For this review, take the finished solid that the model builds, in its own axes (mm). A direction names the side the tool comes from. Give positions to 0.01 mm unless a question says otherwise; leave off trailing zeros. Write each loop counter-clockwise with the first axis right and the second up, starting at its lowest first coordinate (ties: lowest second). Pieces come first, ordered by that corner, then holes. Notation, with made-up numbers: M 70,82 L 110,82 A19 cw 110,99 Z; hole C 57,40 d9. An arc over 180 degrees is marked long. Use one line per item in the form item = value. Start each with the question number.
Q1. Consider section A-A on z = 3.75. Write out the cut boundary in (x, y), and give its area (3 significant figures).
Q2. Tool access review of faces 1 (the cylindrical face through (-12.69, 24.397, 4.162)), 2 (the flat face through (1.05, -37.96, 0.99)), 3 (the cylindrical face through (34.9, -25.8, 1)): name each direction out of +Z, -Z, +X, -X, +Y, -Y from which nothing blocks a thin tool from reaching the whole face with its end or side.
Q3. Consider section C-C on z = 10.25. Write out the cut boundary in (x, y), and give its area (3 significant figures).
Q4. Clearance check with flat-ended pins moving along their axes: pin 1 Ø2.5 at (x, y) = (33.3, -12.68) entering from -Z; pin 2 Ø2 at (x, z) = (30, 1) entering from +Y; pin 3 Ø4 at (y, z) = (-53.5, 2.5) entering from -X; pin 4 Ø4 at (y, z) = (-42, 7) entering from +X. State where each tip first meets the part, or that it passes through.
Q5. Consider section D-D on x = 66.6. Write out the cut boundary in (y, z).
Q6. Consider section B-B on y = 0. Write out the cut boundary in (x, z), and give its area (3 significant figures).
Q7. Mouldability with a two-part tool opening along Y and no side actions: class faces 4 (the flat face through (34, -15, 0)), 5 (the cylindrical face through (28.35, -19.3, 0.99)) as released by +Y, released by -Y, zero draft, split by the parting line, or undercut.
Q8. For probe 1 along Y at (x, z) = (33.3, 1.25); probe 2 along Y at (x, z) = (0, 3.1); probe 3 along X at (y, z) = (-13, 4), list the stretches that pass through material, from the lowest coordinate up. Write a range as [from, to].
```python
from build123d import *

# Parameters (mm, degrees)
SKETCH_1_R          = 30
SKETCH_1_R_2        = 27.5
EXTRUDE_1_DEPTH     = 13
SKETCH_1_R_3        = 29.999999999999996
EXTRUDE_1_2_DEPTH   = 13
EXTRUDE_1_3_DEPTH   = 13
EXTRUDE_2_DEPTH     = 2
SKETCH_3_R          = 1.6500000000000017
SKETCH_3_R_2        = 1.5999999999999979
SKETCH_3_R_3        = 1.5999999999999985
SKETCH_3_R_4        = 1.6000000000000019
CUT_EXTRUDE_5_DEPTH = 132.10250765535577
FILLET_1_R          = 10


with BuildPart() as part:
    # Sketch 1 → Extrude 1 (new body)
    with BuildSketch(Plane.XY):
        with Locations(Location((0, 0, 0), (0, 0, 180))):
            Circle(SKETCH_1_R)
        with Locations(Location((0, 0, 0), (0, 0, 180))):
            Circle(SKETCH_1_R_2, mode=Mode.SUBTRACT)
    extrude(amount=EXTRUDE_1_DEPTH)



with BuildPart() as body_2:
    # Sketch 1 → Extrude 1 2 (new body)
    with BuildSketch(Plane.XY):
        with Locations(Location((66.6, 0, 0), (0, 0, 180))):
            Circle(SKETCH_1_R_3)
        with Locations(Location((66.6, 0, 0), (0, 0, 180))):
            Circle(SKETCH_1_R_2, mode=Mode.SUBTRACT)
    extrude(amount=EXTRUDE_1_2_DEPTH)


with BuildPart() as body_3:
    # Sketch 1 → Extrude 1 3 (new body)
    with BuildSketch(Plane.XY):
        with Locations(Location((33.30000000000001, -57.6772918920436, 0), (0, 0, 180))):
            Circle(SKETCH_1_R_3)
        with Locations(Location((33.30000000000001, -57.6772918920436, 0), (0, 0, 180))):
            Circle(SKETCH_1_R_2, mode=Mode.SUBTRACT)
    extrude(amount=EXTRUDE_1_3_DEPTH)


with BuildPart() as part_1:
    add(part.part)

    add(body_2.part)  # Extrude 2 merges body 2

    add(body_3.part)  # Extrude 2 merges body 3
    # Sketch 2 → Extrude 2 (add)
    with BuildSketch(Plane.XY):
        with BuildLine():
            Line((26.3198925252566, 18.070831312697457), (40.280107474743396, 18.070831312697457))
            ThreePointArc((40.280107474743396, 18.070831312697457), (42.3441853289733, 18.516758123597654), (44.04009212120862, 19.77499826802639))
            ThreePointArc((44.04009212120862, 19.77499826802639), (92.58076211353317, 15), (72.44569692050842, -29.424952464083248))
            ThreePointArc((72.44569692050842, -29.424952464083248), (70.50807559525407, -30.264530756395246), (69.08985272167097, -31.829111208097117))
            Line((69.08985272167097, -31.829111208097117), (62.10974524692759, -43.91901199664395))
            ThreePointArc((62.10974524692759, -43.91901199664395), (61.46389026628078, -45.92951925924603), (61.70560479929982, -48.027337695986766))
            ThreePointArc((61.70560479929982, -48.027337695986766), (33.300000000000004, -87.6772918920436), (4.894395200700185, -48.02733769598677))
            ThreePointArc((4.894395200700185, -48.02733769598677), (5.13610973371921, -45.92951925924604), (4.4902547530724135, -43.91901199664397))
            Line((4.4902547530724135, -43.91901199664397), (-2.489852721670984, -31.829111208097103))
            ThreePointArc((-2.489852721670984, -31.829111208097103), (-3.9080755952540875, -30.264530756395228), (-5.845696920508439, -29.42495246408323))
            ThreePointArc((-5.845696920508439, -29.42495246408323), (-25.980762113533153, 15.000000000000009), (22.55990787879137, 19.77499826802639))
            ThreePointArc((22.55990787879137, 19.77499826802639), (24.25581467102669, 18.516758123597654), (26.3198925252566, 18.070831312697457))
        make_face()
    extrude(amount=EXTRUDE_2_DEPTH)

    # Sketch 3 → Cut-Extrude 5 (cut, through all)
    with BuildSketch(Plane.XY):
        with Locations(Location((33.3, -19.225763964014533, 0), (0, 0, 180))):
            Circle(SKETCH_3_R)
        with Locations(Location((33.3, -12.678793774014526, 0), (0, 0, 180))):
            Circle(SKETCH_3_R_2)
        with Locations(Location((39.84697019, -19.225763964014533, 0), (0, 0, 180))):
            Circle(SKETCH_3_R_3)
        with Locations(Location((33.3, -25.772734154014536, 0), (0, 0, 180))):
            Circle(SKETCH_3_R_3)
        with Locations(Location((26.75302980999999, -19.225763964014533, 0), (0, 0, 180))):
            Circle(SKETCH_3_R_4)
    extrude(amount=CUT_EXTRUDE_5_DEPTH, mode=Mode.SUBTRACT)

    # Fillet 1
    # the kernel refuses this fillet: 10 mm, written as the material it takes off along each edge
    with BuildSketch(Plane(origin=(0, 0, 13), x_dir=(-1, 1.2e-16, 0), z_dir=(1.2e-16, 1, 0))) as fillet_1_piece_1:
        with BuildLine():
            CenterArc((37.5, -6.614378277661482), FILLET_1_R, 138.59037789072914, 41.409622109270856)
            Line((27.5, -6.614378277661482), (27.3, -6.614378277661482))
            Line((27.3, -6.614378277661482), (27.3, 0))
            Line((27.3, 0), (27.5, 0.1999999999999993))
            ThreePointArc((27.5, 0.1999999999999993), (28.75, 0.1999999999999993), (29.85, 0.1322875655532254))
            Line((29.85, 0.1322875655532254), (30, -3.55e-15))
        make_face()
    revolve(axis=Axis((0, 0, 13), (0, 0, 1)), mode=Mode.SUBTRACT)
    with BuildSketch(Plane(origin=(66.6, 0, 13), x_dir=(-1, 1.2e-16, 0), z_dir=(1.2e-16, 1, 0))) as fillet_1_piece_2:
        with BuildLine():
            CenterArc((37.5, -6.614378277661482), FILLET_1_R, 138.59037789072914, 41.409622109270856)
            Line((27.5, -6.614378277661482), (27.299999999999997, -6.614378277661482))
            Line((27.299999999999997, -6.614378277661482), (27.299999999999997, 0))
            Line((27.299999999999997, 0), (27.5, 0.1999999999999993))
            ThreePointArc((27.5, 0.1999999999999993), (28.75, 0.1999999999999993), (29.85, 0.1322875655532254))
            Line((29.85, 0.1322875655532254), (30, -3.55e-15))
        make_face()
    revolve(axis=Axis((66.6, 0, 13), (0, 0, 1)), mode=Mode.SUBTRACT)
    with BuildSketch(Plane(origin=(33.30000000000001, -57.6772918920436, 13), x_dir=(-1, 0, 0), z_dir=(0, 1, 0))) as fillet_1_piece_3:
        with BuildLine():
            CenterArc((37.5, -6.614378277661478), FILLET_1_R, 138.59037789072914, 41.409622109270856)
            Line((27.5, -6.614378277661478), (27.3, -6.614378277661478))
            Line((27.3, -6.614378277661478), (27.3, 0))
            Line((27.3, 0), (27.5, 0.1999999999999993))
            ThreePointArc((27.5, 0.1999999999999993), (28.75, 0.1999999999999993), (29.849999999999998, 0.1322875655532254))
            Line((29.849999999999998, 0.1322875655532254), (30, -3.55e-15))
        make_face()
    revolve(axis=Axis((33.30000000000001, -57.6772918920436, 13), (0, 0, 1)), mode=Mode.SUBTRACT)


solid = part_1.part
```
Working result:
q1.outline = C 0,0 d60; C 33.3,-57.68 d60; C 66.6,0 d60; hole C 0,0 d55; hole C 33.3,-57.68 d55; hole C 66.6,0 d55
q1.area = 1,350 mm²
q2.face_1 = +Z
q2.face_2 = +Z, -Z, -X
q2.face_3 = +Z, -Z
q3.outline = C 0,0 d60; C 33.3,-57.68 d60; C 66.6,0 d60; hole C 0,0 d56.55; hole C 33.3,-57.68 d56.55; hole C 66.6,0 d56.55
q3.area = 946 mm²
q4.pin_1 = through
q4.pin_2 = 18.07
q4.pin_3 = 3.38
q4.pin_4 = 60
q5.outline = M -36.14,0 L 30,0 L 30,13 A10 ccw 27.5,6.39 L 27.5,2 L -27.5,2 L -27.5,6.39 A10 ccw -30,13 L -30,2 L -36.14,2 Z
q6.outline = M -30,0 L 96.6,0 L 96.6,13 A10 ccw 94.1,6.39 L 94.1,2 L 39.1,2 L 39.1,6.39 A10 ccw 36.6,13 L 36.6,2 L 30,2 L 30,13 A10 ccw 27.5,6.39 L 27.5,2 L -27.5,2 L -27.5,6.39 A10 ccw -30,13 Z
q6.area = 342 mm²
q7.face_4 = zero draft
q7.face_5 = undercut
q8.probe_1 = [-87.68, -27.37], [-24.17, -20.88], [-17.58, -14.28], [-11.08, 18.07]
q8.probe_2 = [-30, -27.5], [27.5, 30]
q8.probe_3 = [-27.04, -24.23], [24.23, 27.04], [39.56, 42.37], [90.83, 93.64]
